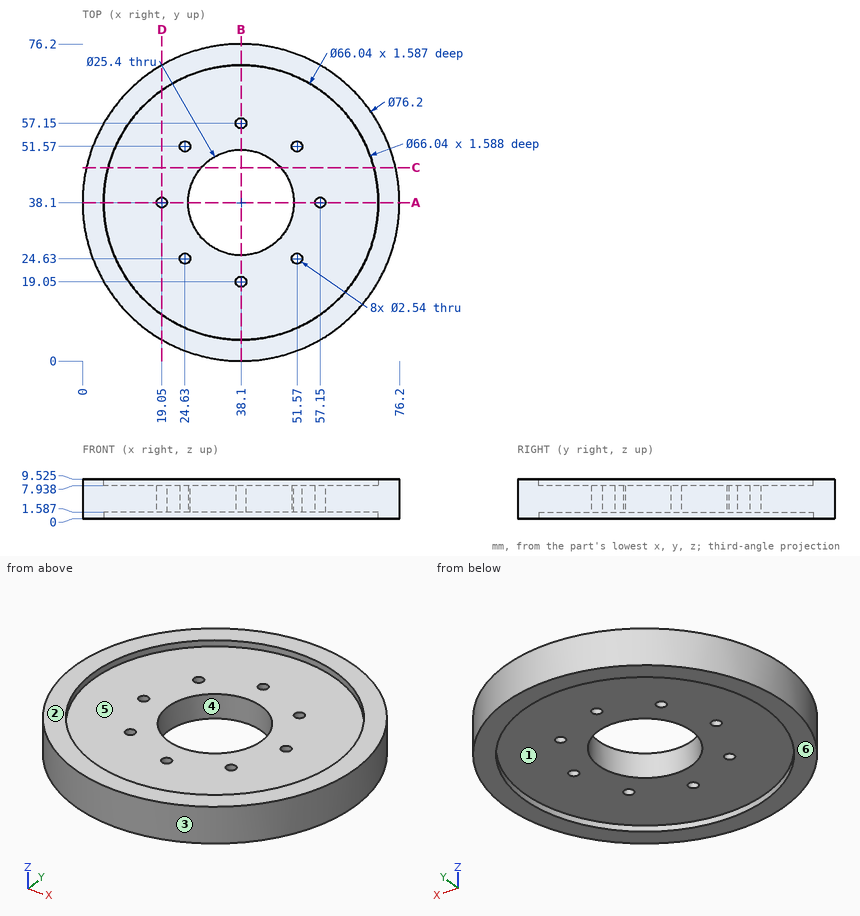
Here's the drawing with two shaded views (mm, measured from the low corner). I have some questions. A direction names the side the tool comes from. Round coordinates to 2 decimals unless told otherwise and drop trailing zeros. Loops run counter-clockwise (first coordinate to the right, second up) from the corner with the lowest first, then second, coordinate; pieces in that order, holes last. Notation, with made-up numbers: (29.25, 46.5) -> (50.25, 46.5) arc R22 ccw to (50.25, 60.5) -> close; hole circle Ø6 at (-10.75, 80.25). An arc over 180 degrees is marked (long way). Answer as CSV lines item,"result". Start each with the question number.
1. Imagine slicing it at A-A on y = 38.1. Write out the boundary of the cut face in (x, z) (1 decimal).
2. I'm going to push flat-ended pins straight in: P1, Ø3.5, axis at x = 51.57, y = 51.57, coming from the -Z side; P2, Ø5, axis at y = 10.5, z = 4.5, coming from the -X side (1 decimal); P3, Ø3, axis at y = 61.5, z = 1, coming from the -X side. Where does each tip first touch, or does it pass through?
3. Imagine slicing it at C-C on y = 46.5. Write out the boundary of the cut face in (x, z) (1 decimal), plus the area to 3 significant figures.
4. If we mould it in two halves opening along Y, with no side actions, what happens to the marked faces 3, 4, 5 and 6? For each: pulls with the +Y half, pulls with the -Y half, needs draft (parallel to the pull), parting line crosses it, or undercut.
5. For the marked faces 1 and 2, which set-ups out of +Z, -Z, +X, -X, +Y, -Y let a thin tool reach every point of the face, with its end or its side?
6. I need wall thicknesses on probe 1 along X at (y, z) = (24.5, 5) (1 decimal); probe 2 along X at (y, z) = (38.5, 7.5) (1 decimal); probe 3 along Z at (x, y) = (24, 56.5). Which ranges of each line are inside material? Lowest first, please. Write a range as from..to.
7. Imagine slicing it at D-D on x = 19.05. Write out the boundary of the cut face in (y, z) (1 decimal), plus the area to 3 significant figures.
Solution:
1,outline,"(0, 0) -> (5.1, 0) -> (5.1, 1.6) -> (17.8, 1.6) -> (17.8, 7.9) -> (5.1, 7.9) -> (5.1, 9.5) -> (0, 9.5) -> close; (20.3, 1.6) -> (25.4, 1.6) -> (25.4, 7.9) -> (20.3, 7.9) -> close; (50.8, 1.6) -> (55.9, 1.6) -> (55.9, 7.9) -> (50.8, 7.9) -> close; (58.4, 1.6) -> (71.1, 1.6) -> (71.1, 0) -> (76.2, 0) -> (76.2, 9.5) -> (71.1, 9.5) -> (71.1, 7.9) -> (58.4, 7.9) -> close"
2,P1,"z = 1.59"
2,P2,"x = 9.4"
2,P3,"x = 6.92"
3,outline,"(0.9, 0) -> (6.2, 0) -> (6.2, 1.6) -> (28.6, 1.6) -> (28.6, 7.9) -> (6.2, 7.9) -> (6.2, 9.5) -> (0.9, 9.5) -> close; (47.6, 1.6) -> (70, 1.6) -> (70, 0) -> (75.3, 0) -> (75.3, 9.5) -> (70, 9.5) -> (70, 7.9) -> (47.6, 7.9) -> close"
3,area,"384 mm²"
4,face 3,"parting line crosses it"
4,face 4,"undercut"
4,face 5,"undercut"
4,face 6,"needs draft"
5,face 1,"-Z"
5,face 2,"+Z, +X, -X, +Y, -Y"
6,probe 1,"2.5..23.4, 25.9..50.3, 52.8..73.7"
6,probe 2,"0..17.8, 20.3..25.4, 50.8..55.9, 58.4..76.2"
6,probe 3,"1.59..7.94"
7,outline,"(5.1, 0) -> (11.1, 0) -> (11.1, 1.6) -> (36.8, 1.6) -> (36.8, 7.9) -> (11.1, 7.9) -> (11.1, 9.5) -> (5.1, 9.5) -> close; (39.4, 1.6) -> (65.1, 1.6) -> (65.1, 0) -> (71.1, 0) -> (71.1, 9.5) -> (65.1, 9.5) -> (65.1, 7.9) -> (39.4, 7.9) -> close"
7,area,"441 mm²"
